Could you check a few things on this drawing? It's one solid part, dimensions in mm from its lowest x, y, z. A direction names the side the tool comes from. Give positions to 0.01 mm unless a question says otherwise; leave off trailing zeros. Loops run counter-clockwise (first coordinate to the right, second up) from the corner with the lowest first, then second, coordinate; pieces in that order, holes last.
1. Imagine slicing it at A-A (z = 11.25). List the corners of the cut face in (x, y) for me.
2. Imagine slicing it at B-B (x = 18). List the corners of the cut face in (y, z) for me, plus the area to 3 significant figures.
3. Imagine slicing it at D-D (x = 46.5). List the corners of the cut face in (y, z) for me.
4. I need wall thicknesses on line 1 along Z through (x, y) = (55.5, 32); line 2 along Y through (x, z) = (21.5, 6.75); line 3 along X through (y, z) = (46, 11.5). Which ranges of each line are inside material? Lowest first, please.
5. Imagine slicing it at C-C (y = 24). List the corners of the cut face in (x, z) for me.
6. For the marked faces 1, 2 and 3, which set-ups out of +Z, -Z, +X, -X, +Y, -Y let a thin tool reach every point of the face, with its end or its side?
7. For P1, Ø1.6, axis at x = 42.5, z = 11, coming from the +Y side; P2, Ø10, axis at y = 37.5, z = 8, coming from the -X side; P3, Ø2.5, axis at x = 42, z = 11.5, coming from the -Y side, each with a flat end and sliding along its axis, tell me the tip position at first contact or that it passes through.
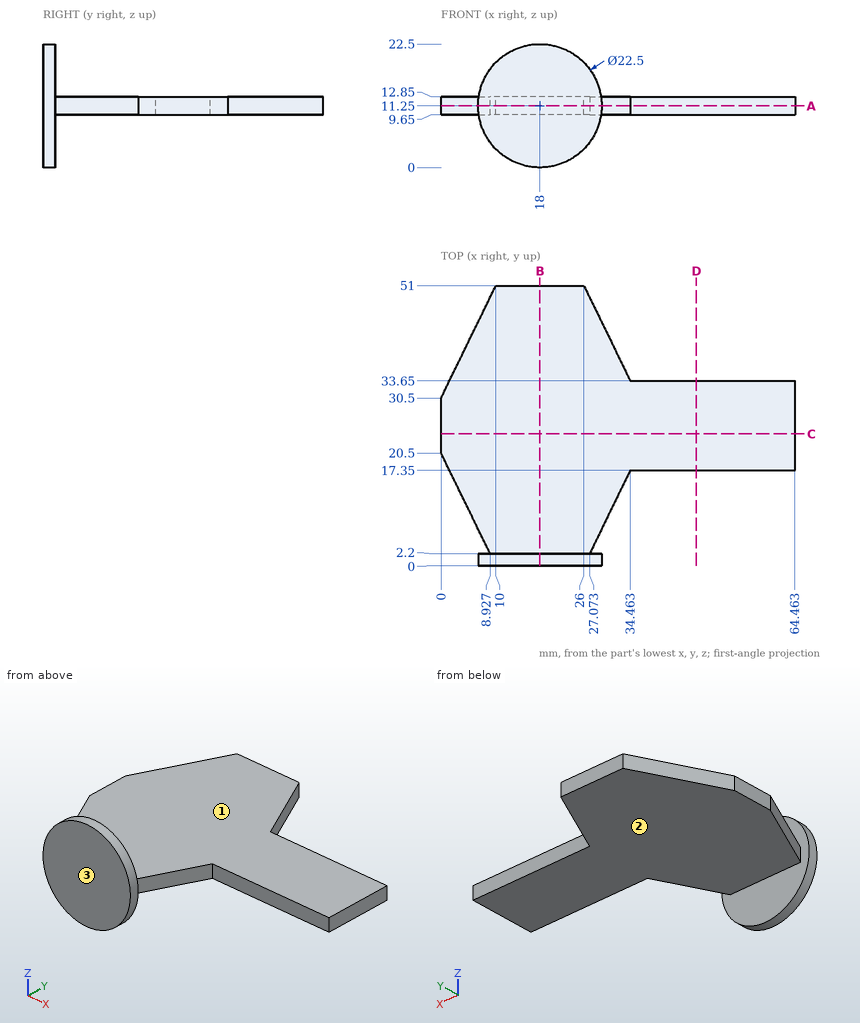
Derived:
1. outline: (0, 20.5) - (8.93, 2.2) - (6.75, 2.2) - (6.75, 0) - (29.25, 0) - (29.25, 2.2) - (27.07, 2.2) - (34.46, 17.35) - (64.46, 17.35) - (64.46, 33.65) - (34.46, 33.65) - (26, 51) - (10, 51) - (0, 30.5) - close
2. outline: (0, 0) - (2.2, 0) - (2.2, 9.65) - (51, 9.65) - (51, 12.85) - (2.2, 12.85) - (2.2, 22.5) - (0, 22.5) - close
2. area: 206 mm2
3. outline: (17.35, 9.65) - (33.65, 9.65) - (33.65, 12.85) - (17.35, 12.85) - close
4. line 1: z = 9.65 to 12.85
4. line 2: y = 0 to 2.2
4. line 3: x = 7.56 to 28.44
5. outline: (0, 9.65) - (64.46, 9.65) - (64.46, 12.85) - (0, 12.85) - close
6. face 1: +Z, +X, -X, +Y
6. face 2: -Z, +X, -X, +Y
6. face 3: +Z, -Z, +X, -X, -Y
7. P1: stops at y = 33.65
7. P2: stops at x = 1.11
7. P3: stops at y = 17.35
